from build123d import *

# Parameters (mm, degrees)
F1_DEPTH    = 5
F3_T1_DEPTH = 5
F3_T3_DEPTH = 5
F4_T1_DEPTH = 6.2324692544
F4_T3_DEPTH = 6.2324692544
F2_R        = 1.65
F5_DEPTH    = 8.001
F6_SIZE     = 0.5


# Not quite as in the source:
# - a fillet or chamfer that OpenCascade refuses, or shapes differently, is made with other operations: its cross-section is extruded or revolved along the edge and cut away or added
# - a pattern or mirror of a feature is missing from the dataset's text; its kind, count and spacing are read off the source's solid


with BuildPart() as f1:
    # F0 (on Front) → F1 (new body, symmetric)
    with BuildSketch(Plane.XZ):
        with BuildLine():
            Line((23.5, -9), (23.5, -1))
            Line((23.5, -1), (4.8989794856, -1))
            ThreePointArc((4.8989794856, -1), (3.1622776602, -3.8729833462), (0, -5))
            ThreePointArc((0, -5), (-3.1622776602, -3.8729833462), (-4.8989794856, -1))
            Line((-4.8989794856, -1), (-23.5, -1))
            Line((-23.5, -1), (-23.5, -9))
            Line((-23.5, -9), (-16.5, -9))
            Line((-16.5, -9), (-16.5, -4))
            Line((-16.5, -4), (-6.9282032303, -4))
            ThreePointArc((-6.9282032303, -4), (-4, -6.9282032303), (0, -8))
            ThreePointArc((0, -8), (4, -6.9282032303), (6.9282032303, -4))
            Line((6.9282032303, -4), (16.5, -4))
            Line((16.5, -4), (16.5, -9))
            Line((16.5, -9), (23.5, -9))
        make_face()
    extrude(amount=F1_DEPTH, both=True)

    # F3: fillet of radius 7 on 8 edges, made by hand

    # F3_s2 → F3_t1 (join)
    with BuildSketch(Plane.XZ.offset(-5)):
        with BuildLine():
            ThreePointArc((9.7917960675, -4), (13.9750962002, -5.3875139198), (16.5, -9))
            Line((16.5, -9), (16.5, -4))
            Line((16.5, -4), (9.7917960675, -4))
        make_face()
        with BuildLine():
            ThreePointArc((5.4389541478, -5.8666666667), (7.6420004255, -4.4833546462), (10.1980390272, -4))
            Line((10.1980390272, -4), (6.9282032303, -4))
            ThreePointArc((6.9282032303, -4), (6.2536194731, -4.989212712), (5.4389541478, -5.8666666667))
        make_face()
        with BuildLine():
            ThreePointArc((-9.7917960675, -4), (-13.9750962002, -5.3875139198), (-16.5, -9))
            Line((-16.5, -9), (-16.5, -4))
            Line((-16.5, -4), (-9.7917960675, -4))
        make_face()
        with BuildLine():
            ThreePointArc((-5.4389541478, -5.8666666667), (-7.6420004255, -4.4833546462), (-10.1980390272, -4))
            Line((-10.1980390272, -4), (-6.9282032303, -4))
            ThreePointArc((-6.9282032303, -4), (-6.2536194731, -4.989212712), (-5.4389541478, -5.8666666667))
        make_face()
    extrude(amount=F3_T1_DEPTH)

    # F3_s4 → F3_t3 (join)
    with BuildSketch(Plane.XZ):
        with BuildLine():
            ThreePointArc((9.7917960675, -4), (13.9750962002, -5.3875139198), (16.5, -9))
            Line((16.5, -9), (16.5, -4))
            Line((16.5, -4), (9.7917960675, -4))
        make_face()
        with BuildLine():
            ThreePointArc((5.4389541478, -5.8666666667), (7.6420004255, -4.4833546462), (10.1980390272, -4))
            Line((10.1980390272, -4), (6.9282032303, -4))
            ThreePointArc((6.9282032303, -4), (6.2536194731, -4.989212712), (5.4389541478, -5.8666666667))
        make_face()
        with BuildLine():
            ThreePointArc((-9.7917960675, -4), (-13.9750962002, -5.3875139198), (-16.5, -9))
            Line((-16.5, -9), (-16.5, -4))
            Line((-16.5, -4), (-9.7917960675, -4))
        make_face()
        with BuildLine():
            ThreePointArc((-5.4389541478, -5.8666666667), (-7.6420004255, -4.4833546462), (-10.1980390272, -4))
            Line((-10.1980390272, -4), (-6.9282032303, -4))
            ThreePointArc((-6.9282032303, -4), (-6.2536194731, -4.989212712), (-5.4389541478, -5.8666666667))
        make_face()
    extrude(amount=F3_T3_DEPTH)

    # F4: chamfer of 0.5 on 4 edges, made by hand

    # F4_s2 → F4_t1 (cut)
    with BuildSketch(Plane.XZ.offset(-6.2324692544)):
        with BuildLine():
            Line((-4.7731743681, -1.4483837223), (-5.3918225964, -0.9880608955))
            Line((-5.3918225964, -0.9880608955), (-5.3918225964, -0.9780608955))
            ThreePointArc((-5.3918225964, -0.9780608955), (-5.145401041, -0.99), (-4.8989794856, -0.99))
            Line((-4.8989794856, -0.99), (-4.8891815266, -0.998))
            ThreePointArc((-4.8891815266, -0.998), (-4.8374189809, -1.2245315852), (-4.7635959284, -1.445510833))
            Line((-4.7635959284, -1.445510833), (-4.7731743681, -1.4483837223))
        make_face()
        with BuildLine():
            Line((5.3918225964, -0.9880608955), (4.7731743681, -1.4483837223))
            Line((4.7731743681, -1.4483837223), (4.7635959284, -1.445510833))
            ThreePointArc((4.7635959284, -1.445510833), (4.8374189809, -1.2245315852), (4.8891815266, -0.998))
            Line((4.8891815266, -0.998), (4.8989794856, -0.99))
            ThreePointArc((4.8989794856, -0.99), (5.145401041, -0.99), (5.3918225964, -0.9780608955))
            Line((5.3918225964, -0.9780608955), (5.3918225964, -0.9880608955))
        make_face()
    extrude(amount=F4_T1_DEPTH, mode=Mode.SUBTRACT)

    # F4_s4 → F4_t3 (cut)
    with BuildSketch(Plane.XZ):
        with BuildLine():
            Line((-4.7731743681, -1.4483837223), (-5.3918225964, -0.9880608955))
            Line((-5.3918225964, -0.9880608955), (-5.3918225964, -0.9780608955))
            ThreePointArc((-5.3918225964, -0.9780608955), (-5.145401041, -0.99), (-4.8989794856, -0.99))
            Line((-4.8989794856, -0.99), (-4.8891815266, -0.998))
            ThreePointArc((-4.8891815266, -0.998), (-4.8374189809, -1.2245315852), (-4.7635959284, -1.445510833))
            Line((-4.7635959284, -1.445510833), (-4.7731743681, -1.4483837223))
        make_face()
        with BuildLine():
            Line((5.3918225964, -0.9880608955), (4.7731743681, -1.4483837223))
            Line((4.7731743681, -1.4483837223), (4.7635959284, -1.445510833))
            ThreePointArc((4.7635959284, -1.445510833), (4.8374189809, -1.2245315852), (4.8891815266, -0.998))
            Line((4.8891815266, -0.998), (4.8989794856, -0.99))
            ThreePointArc((4.8989794856, -0.99), (5.145401041, -0.99), (5.3918225964, -0.9780608955))
            Line((5.3918225964, -0.9780608955), (5.3918225964, -0.9880608955))
        make_face()
    extrude(amount=F4_T3_DEPTH, mode=Mode.SUBTRACT)

    # F2 (on face) → F5 (cut, through all)
    with BuildSketch(Plane(origin=(0, 0, -9), x_dir=(1, 0, 0), z_dir=(0, 0, -1))):
        with Locations((19.5, 0)):
            Circle(F2_R)
    f5 = extrude(amount=-F5_DEPTH, mode=Mode.SUBTRACT)

    # F5_copies: F5 across plane
    add(f5.mirror(Plane(origin=(0, 0, 0), x_dir=(0, 0, -1), z_dir=(-1, 0, 0))), mode=Mode.SUBTRACT)

    # F6
    f6_edges = [f1.edges().sort_by_distance(p)[0] for p in [
        (19.5, 1.65, -9),
        (19.5, -1.65, -9),
        (19.5, 1.65, -1),
        (-19.5, 1.65, -9),
        (-19.5, 1.65, -1),
        (-19.5, -1.65, -9),
        (-19.5, -1.65, -1),
        (19.5, -1.65, -1),
    ]]
    chamfer(f6_edges, length=F6_SIZE)


solid = f1.part
Verification items for the finished model (mm, model axes). A direction names the side the tool comes from. Round coordinates to 2 decimals unless told otherwise and drop trailing zeros. Loops run counter-clockwise (first coordinate to the right, second up) from the corner with the lowest first, then second, coordinate; pieces in that order, holes last. Notation, with made-up numbers: (56.25, 82) - (96.25, 82) arc R21 ccw to (96.25, 95) - close; hole circle Ø9 at (-36.75, 33). An arc over 180 degrees is marked (long way). Answer in a Markdown table with one row per item. Add a question column.
Q1. Section check C-C on y = -3.25. Enter the section's corners in (x, z).
Q2. Section check A-A on x = 19.5. Enter the section's corners in (y, z).
Q3. Section check D-D on z = -6.5. Enter the section's corners in (x, y).
Q4. Material ranges on line 1 (Y direction, x = -19.5, z = -5); line 2 (X direction, y = 0, z = -6.5); line 3 (X direction, y = 4, z = -6), recorded low to high.
Q5. Tool access check on faces 1 (the face through (-7.515, 0.07, -4.535)), 2 (the face through (0, -5, -6)). Record the directions out of +Z, -Z, +X, -X, +Y, -Y that give a thin tool (end or side, any length) a straight path to the whole face; none if there is none.
Q6. Section check B-B on y = 0. State how many separate pieces and enclosed holes the cut face has, plus the area to 3 significant figures.
Q7. Release check for a two-part mould opening along Y. For faces 3 (the face through (18.19, 1, -5.05)), 4 (the face through (0, 5, -6)), 5 (the face through (-18.19, 1, -5.05)), 6 (the face through (-14.007, 0.07, -5.412)) record: pulls with the +Y half, pulls with the -Y half, needs draft (parallel to the pull), parting line crosses it, or undercut.
Found:
| question | item | result |
|---|---|---|
| 1 | outline | (-23.5, -9) - (-16.5, -9) arc R7 cw to (-9.99, -4) arc R7 cw to (-5.44, -5.87) arc R8 ccw to (5.44, -5.87) arc R7 cw to (9.99, -4) arc R7 cw to (16.5, -9) - (23.5, -9) - (23.5, -1) - (5.38, -1) - (4.79, -1.44) arc R5 cw to (-4.79, -1.44) - (-5.38, -1) - (-23.5, -1) - close |
| 2 | outline | (-5, -9) - (-2.15, -9) - (-1.65, -8.5) - (-1.65, -1.5) - (-2.15, -1) - (-5, -1) - close; (1.65, -8.5) - (2.15, -9) - (5, -9) - (5, -1) - (2.15, -1) - (1.65, -1.5) - close |
| 3 | outline | (-23.5, -5) - (-15.15, -5) - (-15.15, 5) - (-23.5, 5) - close; (-4.66, -5) - (4.66, -5) - (4.66, 5) - (-4.66, 5) - close; (15.15, -5) - (23.5, -5) - (23.5, 5) - (15.15, 5) - close; hole circle Ø3.3 at (-19.5, 0); hole circle Ø3.3 at (19.5, 0) |
| 4 | line 1 | y = -5 to -1.65, 1.65 to 5 |
| 4 | line 2 | x = -23.5 to -21.15, -17.85 to -15.15, -4.66 to 4.66, 15.15 to 17.85, 21.15 to 23.5 |
| 4 | line 3 | x = -23.5 to -14.69, -5.29 to 5.29, 14.69 to 23.5 |
| 5 | face 1 | -Z, +Y, -Y |
| 5 | face 2 | +Z, -Z, +X, -X, -Y |
| 6 | separate pieces | 3 |
| 6 | enclosed holes | 0 |
| 6 | area | 187 mm² |
| 7 | face 3 | undercut |
| 7 | face 4 | pulls with the +Y half |
| 7 | face 5 | undercut |
| 7 | face 6 | needs draft |
